Can you work these out from the model? Positions are in its coordinate system, mm. Give positions to 0.01 mm unless a question says otherwise; leave off trailing zeros. Order: outer loops, then holes, each group sorted by start corner. A loop starts at its lowest first (then second) coordinate and runs counter-clockwise, first axis right, second up. Notation, with made-up numbers: (-35, -26) - (19, -26) arc R13 ccw to (19, -6) - close; hole circle Ø4 at (-35.75, -38). An arc over 180 degrees is marked (long way). Write each question's results on one line, items separated by ' | '. Start each with the question number.
from build123d import *

# Parameters (mm, degrees)
SKETCH2_R           = 100
BOSS_EXTRUDE1_DEPTH = 5
SKETCH3_W           = 0.5
SKETCH3_H           = 20
CUT_EXTRUDE1_DEPTH  = 142.509716981


with BuildPart() as part:
    # Sketch2 → Boss-Extrude1 (new body)
    with BuildSketch(Plane(origin=(0, 0, 0), x_dir=(1, 0, 0), z_dir=(0, 1, 0))):
        with Locations(Location((0, 0, 0), (0, 0, 270))):
            Circle(SKETCH2_R)
    extrude(amount=BOSS_EXTRUDE1_DEPTH)

    # Sketch3 → Cut-Extrude1 (cut, through all)
    with BuildSketch(Plane(origin=(0, 5, 0), x_dir=(1, 0, 0), z_dir=(0, 1, 0))):
        with Locations((-7.5, 75)):
            Rectangle(SKETCH3_W, SKETCH3_H)
        with Locations((7.5, 75)):
            Rectangle(SKETCH3_W, SKETCH3_H)
        Polygon((60.166651246, -25.788303121), (77.487159322, -35.788303121), (77.237159322, -36.221315823), (59.916651246, -26.221315823), align=None)
        Polygon((52.666651246, -38.778684177), (69.987159322, -48.778684177), (69.737159322, -49.211696879), (52.416651246, -39.211696879), align=None)
        Polygon((-52.416651246, -39.211696879), (-69.737159322, -49.211696879), (-69.987159322, -48.778684177), (-52.666651246, -38.778684177), align=None)
        Polygon((-59.916651246, -26.221315823), (-77.237159322, -36.221315823), (-77.487159322, -35.788303121), (-60.166651246, -25.788303121), align=None)
    extrude(amount=-CUT_EXTRUDE1_DEPTH, mode=Mode.SUBTRACT)

    # Sketch7 → Ø10.0mm Dowel Hole1 (revolve, cut)
    with BuildSketch(Plane(origin=(0, 0, 0), x_dir=(0, 0, -1), z_dir=(1, 0, 0))):
        Polygon((0, 0), (0, 5), (5, 5), (5, 0.025), (5.025, 0), align=None)
    revolve(axis=Axis((0, -6.35, 0), (0, 1, 0)), mode=Mode.SUBTRACT)


solid = part.part
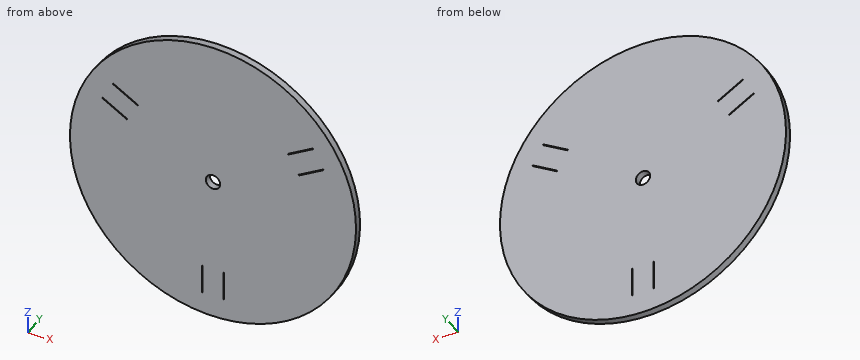
Q1. If we section it at C-C (x = 0): Please give me the cut outline in (y, z) (3 decimals), plus the area to 3 significant figures.
Q2. Will these pins go through, and if not, where does the flat tip stop? P1, Ø0.6, axis at x = -7.5, y = 1.5, coming from the +Z side; P2, Ø1, axis at y = 3.5, z = 18.5, coming from the +X side; P3, Ø3, axis at x = 7, y = 2, coming from the -Z side.
Q3. If I drill on probe 1 along X at (y, z) = (1.85, 0); probe 2 along X at (y, z) = (1.1, -78); probe 3 along X at (y, z) = (1.1, 39), over which ranges is the centre line in solid material (lowest first)? Write a range as from..to.
Q4. If we section it at A-A (y = 0.95): Please give me the cut outline in (x, z).
Q5. If we section it at D-D (z = 33): Please give me the cut outline in (x, y), plus the area to 3 significant figures.
Q6. If we section it at B-B (z = 0): Please give me the cut outline in (x, y) (3 decimals).
Findings below:
1) outline: (0, -100) - (5, -100) - (5, -5) - (0.025, -5) - (0, -5.025) - close; (0, 5.025) - (0.025, 5) - (5, 5) - (5, 100) - (0, 100) - close | area: 950 mm2
2) P1: stops at z = 99.74 | P2: stops at x = 98.37 | P3: stops at z = -99.85
3) probe 1: x = -100..-5, 5..100 | probe 2: x = -62.58..-7.75, -7.25..7.25, 7.75..62.58 | probe 3: x = -92.08..-53.05, -52.54..52.54, 53.05..92.08
4) outline: circle Ø200 at (0, 0); hole (-77.49, 35.79) - (-60.17, 25.79) - (-59.92, 26.22) - (-77.24, 36.22) - close; hole (-69.99, 48.78) - (-52.67, 38.78) - (-52.42, 39.21) - (-69.74, 49.21) - close; hole (-7.75, -85) - (-7.25, -85) - (-7.25, -65) - (-7.75, -65) - close; hole circle Ø10 at (0, 0); hole (7.25, -85) - (7.75, -85) - (7.75, -65) - (7.25, -65) - close; hole (52.42, 39.21) - (52.67, 38.78) - (69.99, 48.78) - (69.74, 49.21) - close; hole (59.92, 26.22) - (60.17, 25.79) - (77.49, 35.79) - (77.24, 36.22) - close
5) outline: (-94.4, 0) - (-72.66, 0) - (-72.66, 5) - (-94.4, 5) - close; (-71.66, 0) - (71.66, 0) - (71.66, 5) - (-71.66, 5) - close; (72.66, 0) - (94.4, 0) - (94.4, 5) - (72.66, 5) - close | area: 934 mm2
6) outline: (-100, 0) - (-5.025, 0) - (-5, 0.025) - (-5, 5) - (-100, 5) - close; (5, 0.025) - (5.025, 0) - (100, 0) - (100, 5) - (5, 5) - close
